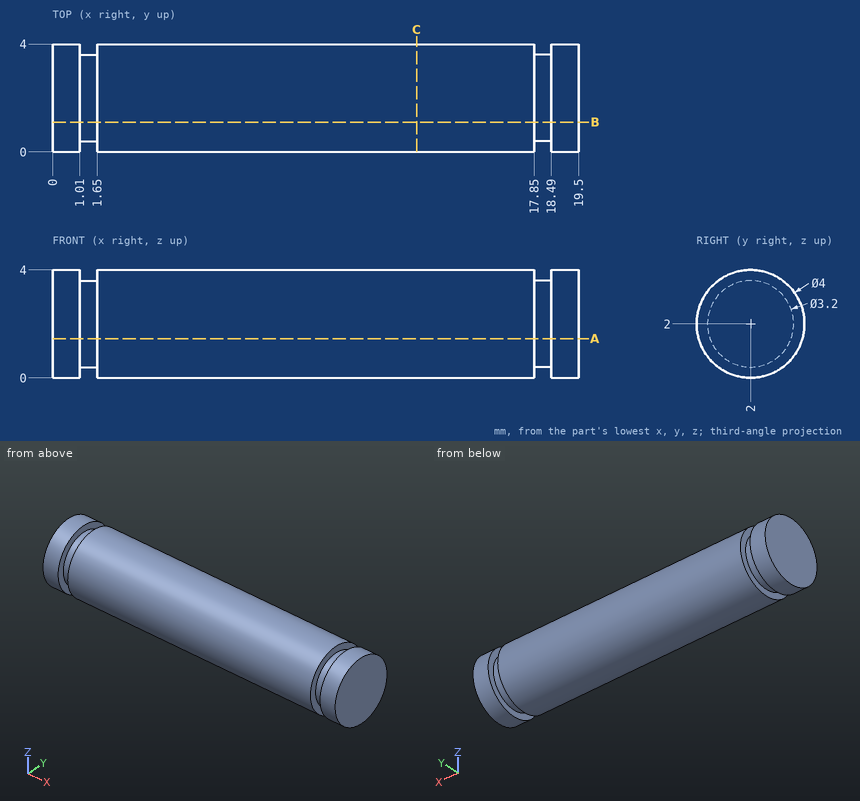
Geometry check sheet. Reference: drawing and pictorial views, mm from the part's lowest x, y, z. Round coordinates to 2 decimals unless told otherwise and drop trailing zeros. Loops run counter-clockwise (first coordinate to the right, second up) from the corner with the lowest first, then second, coordinate; pieces in that order, holes last. Notation, with made-up numbers: (-11.75, 75.25) - (43.25, 75.25) arc R5 cw to (43.25, 80.25) - close; hole circle Ø1 at (-19.75, -39.75). An arc over 180 degrees is marked (long way). Answer as CSV lines item,"result".
(1) Material ranges on line 1 along X through (y, z) = (2.8, 3.55); line 2 along Z through (x, y) = (10, 3.2); line 3 along Z through (x, y) = (7.5, 2.2), recorded low to high.
Output values:
line 1,"x = 0 to 1.01, 1.65 to 17.85, 18.49 to 19.5"
line 2,"z = 0.4 to 3.6"
line 3,"z = 0.01 to 3.99"
(2) Depth check by flat-ended pin: pin 1 Ø1 at (x, z) = (5.5, 0.5) entering from +Y; pin 2 Ø1.2 at (y, z) = (1, 1) entering from -X; pin 3 Ø1.5 at (x, z) = (16, 0.5) entering from -Y. Enter the tip coordinate at first touch or a pass-through.
Output values:
pin 1,"stops at y = 3.73"
pin 2,"stops at x = 0"
pin 3,"stops at y = 0.15"
(3) Cross-section at C-C, the plane x = 13.5. Enter the section's corners in (y, z), and give its area (3 significant figures).
Output values:
outline,"circle Ø4 at (2, 2)"
area,"12.6 mm²"
(4) Cross-section at A-A, the plane z = 1.45. Enter the section's corners in (x, y), and give its area (3 significant figures).
Output values:
outline,"(0, 0.08) - (1.01, 0.08) - (1.01, 0.5) - (1.65, 0.5) - (1.65, 0.08) - (17.85, 0.08) - (17.85, 0.5) - (18.49, 0.5) - (18.49, 0.08) - (19.5, 0.08) - (19.5, 3.92) - (18.49, 3.92) - (18.49, 3.5) - (17.85, 3.5) - (17.85, 3.92) - (1.65, 3.92) - (1.65, 3.5) - (1.01, 3.5) - (1.01, 3.92) - (0, 3.92) - close"
area,"73.9 mm²"
(5) Cross-section at B-B, the plane y = 1.1. Enter the section's corners in (x, z).
Output values:
outline,"(0, 0.21) - (1.01, 0.21) - (1.01, 0.68) - (1.65, 0.68) - (1.65, 0.21) - (17.85, 0.21) - (17.85, 0.68) - (18.49, 0.68) - (18.49, 0.21) - (19.5, 0.21) - (19.5, 3.79) - (18.49, 3.79) - (18.49, 3.32) - (17.85, 3.32) - (17.85, 3.79) - (1.65, 3.79) - (1.65, 3.32) - (1.01, 3.32) - (1.01, 3.79) - (0, 3.79) - close"
